Check sheet for the modelled part. Datum: model origin and axes. Units: mm. Face numbers are marked on the shaded views. A direction names the side the tool comes from. Give positions to 0.01 mm unless a question says otherwise; leave off trailing zeros. Order: outer loops, then holes, each group sorted by start corner. A loop starts at its lowest first (then second) coordinate and runs counter-clockwise, first axis right, second up. Notation, with made-up numbers: (-21, 35.5) - (-9, 35.5) arc R12 ccw to (-9, 52.5) - close; hole circle Ø4 at (58, 47). An arc over 180 degrees is marked (long way). Answer in a Markdown table with one row per item.
from build123d import *

# Parameters (mm, degrees)
SKETCH1_R           = 1.5
BOSS_EXTRUDE1_DEPTH = 3


with BuildPart() as part:
    # Sketch1 → Boss-Extrude1 (new body)
    with BuildSketch(Plane(origin=(0, 0, 0), x_dir=(1, 0, 0), z_dir=(0, 1, 0))):
        with BuildLine():
            Line((20.893657446, 4), (2.081641936, 4))
            ThreePointArc((2.081641936, 4), (2.861028333, 4.588201733), (3.521749436, 5.30713988))
            ThreePointArc((3.521749436, 5.30713988), (3.405395609, 5.596745198), (3.282888305, 5.883801663))
            ThreePointArc((3.282888305, 5.883801663), (1.93527598, 5.894040025), (0.627094961, 5.57027124))
            ThreePointArc((0.627094961, 5.57027124), (0.366286148, 6.046375), (0.084372603, 6.510293938))
            ThreePointArc((0.084372603, 6.510293938), (1.018855105, 7.48132754), (1.683794586, 8.65351323))
            ThreePointArc((1.683794586, 8.65351323), (1.496450048, 8.903135899), (1.303821399, 9.148703928))
            ThreePointArc((1.303821399, 9.148703928), (-0.000522033, 8.809805691), (-1.180330337, 8.158486898))
            ThreePointArc((-1.180330337, 8.158486898), (-1.555477026, 8.550865528), (-1.947855656, 8.926012217))
            ThreePointArc((-1.947855656, 8.926012217), (-1.296536862, 10.105820521), (-0.957638625, 11.410163953))
            ThreePointArc((-0.957638625, 11.410163953), (-1.203206655, 11.602792602), (-1.452829324, 11.79013714))
            ThreePointArc((-1.452829324, 11.79013714), (-2.625015014, 11.125197659), (-3.596048616, 10.190715157))
            ThreePointArc((-3.596048616, 10.190715157), (-4.059967554, 10.472628702), (-4.536071314, 10.733437515))
            ThreePointArc((-4.536071314, 10.733437515), (-4.212302529, 12.041618533), (-4.222540891, 13.389230859))
            ThreePointArc((-4.222540891, 13.389230859), (-4.509597355, 13.511738163), (-4.799202674, 13.62809199))
            ThreePointArc((-4.799202674, 13.62809199), (-5.759348103, 12.682425791), (-6.455432668, 11.528463019))
            ThreePointArc((-6.455432668, 11.528463019), (-6.976508546, 11.680699536), (-7.503891752, 11.809396783))
            ThreePointArc((-7.503891752, 11.809396783), (-7.529737283, 13.156800143), (-7.888414517, 14.455843809))
            ThreePointArc((-7.888414517, 14.455843809), (-8.197396993, 14.499881098), (-8.507248835, 14.537314892))
            ThreePointArc((-8.507248835, 14.537314892), (-9.18992168, 13.375367565), (-9.563620196, 12.080565177))
            ThreePointArc((-9.563620196, 12.080565177), (-10.106342554, 12.09275), (-10.649064912, 12.080565177))
            ThreePointArc((-10.649064912, 12.080565177), (-11.022763428, 13.375367565), (-11.705436272, 14.537314892))
            ThreePointArc((-11.705436272, 14.537314892), (-12.015288115, 14.499881098), (-12.324270591, 14.455843809))
            ThreePointArc((-12.324270591, 14.455843809), (-12.682947825, 13.156800143), (-12.708793355, 11.809396783))
            ThreePointArc((-12.708793355, 11.809396783), (-13.236176561, 11.680699536), (-13.757252439, 11.528463019))
            ThreePointArc((-13.757252439, 11.528463019), (-14.453337005, 12.682425791), (-15.413482434, 13.62809199))
            ThreePointArc((-15.413482434, 13.62809199), (-15.703087752, 13.511738163), (-15.990144217, 13.389230859))
            ThreePointArc((-15.990144217, 13.389230859), (-16.000382579, 12.041618533), (-15.676613793, 10.733437515))
            ThreePointArc((-15.676613793, 10.733437515), (-16.152717554, 10.472628702), (-16.616636492, 10.190715157))
            ThreePointArc((-16.616636492, 10.190715157), (-17.587670094, 11.125197659), (-18.759855783, 11.79013714))
            ThreePointArc((-18.759855783, 11.79013714), (-19.009478453, 11.602792602), (-19.255046482, 11.410163953))
            ThreePointArc((-19.255046482, 11.410163953), (-18.916148245, 10.105820521), (-18.264829452, 8.926012217))
            ThreePointArc((-18.264829452, 8.926012217), (-18.657208082, 8.550865528), (-19.032354771, 8.158486898))
            ThreePointArc((-19.032354771, 8.158486898), (-20.212163074, 8.809805691), (-21.516506507, 9.148703928))
            ThreePointArc((-21.516506507, 9.148703928), (-21.709135156, 8.903135899), (-21.896479694, 8.65351323))
            ThreePointArc((-21.896479694, 8.65351323), (-21.231540213, 7.48132754), (-20.297057711, 6.510293938))
            ThreePointArc((-20.297057711, 6.510293938), (-20.578971255, 6.046375), (-20.839780068, 5.57027124))
            ThreePointArc((-20.839780068, 5.57027124), (-22.147961087, 5.894040025), (-23.495573413, 5.883801663))
            ThreePointArc((-23.495573413, 5.883801663), (-23.618080717, 5.596745198), (-23.734434544, 5.30713988))
            ThreePointArc((-23.734434544, 5.30713988), (-22.788768345, 4.346994451), (-21.634805572, 3.650909885))
            ThreePointArc((-21.634805572, 3.650909885), (-21.78704209, 3.129834008), (-21.915739337, 2.602450802))
            ThreePointArc((-21.915739337, 2.602450802), (-23.263142697, 2.576605271), (-24.562186363, 2.217928037))
            ThreePointArc((-24.562186363, 2.217928037), (-24.606223651, 1.908945561), (-24.643657446, 1.599093719))
            ThreePointArc((-24.643657446, 1.599093719), (-23.481710119, 0.916420874), (-22.186907731, 0.542722358))
            ThreePointArc((-22.186907731, 0.542722358), (-22.199092554, 0), (-22.186907731, -0.542722358))
            ThreePointArc((-22.186907731, -0.542722358), (-23.481710119, -0.916420874), (-24.643657446, -1.599093719))
            ThreePointArc((-24.643657446, -1.599093719), (-24.606223651, -1.908945561), (-24.562186363, -2.217928037))
            ThreePointArc((-24.562186363, -2.217928037), (-23.263142697, -2.576605271), (-21.915739337, -2.602450802))
            ThreePointArc((-21.915739337, -2.602450802), (-21.78704209, -3.129834008), (-21.634805572, -3.650909885))
            ThreePointArc((-21.634805572, -3.650909885), (-22.788768345, -4.346994451), (-23.734434544, -5.30713988))
            ThreePointArc((-23.734434544, -5.30713988), (-23.618080717, -5.596745198), (-23.495573413, -5.883801663))
            ThreePointArc((-23.495573413, -5.883801663), (-22.147961087, -5.894040025), (-20.839780068, -5.57027124))
            ThreePointArc((-20.839780068, -5.57027124), (-20.578971255, -6.046375), (-20.297057711, -6.510293938))
            ThreePointArc((-20.297057711, -6.510293938), (-21.231540213, -7.48132754), (-21.896479694, -8.65351323))
            ThreePointArc((-21.896479694, -8.65351323), (-21.709135156, -8.903135899), (-21.516506507, -9.148703928))
            ThreePointArc((-21.516506507, -9.148703928), (-20.212163074, -8.809805691), (-19.032354771, -8.158486898))
            ThreePointArc((-19.032354771, -8.158486898), (-18.657208082, -8.550865528), (-18.264829452, -8.926012217))
            ThreePointArc((-18.264829452, -8.926012217), (-18.916148245, -10.105820521), (-19.255046482, -11.410163953))
            ThreePointArc((-19.255046482, -11.410163953), (-19.009478453, -11.602792602), (-18.759855783, -11.79013714))
            ThreePointArc((-18.759855783, -11.79013714), (-17.587670094, -11.125197659), (-16.616636492, -10.190715157))
            ThreePointArc((-16.616636492, -10.190715157), (-16.152717554, -10.472628702), (-15.676613793, -10.733437515))
            ThreePointArc((-15.676613793, -10.733437515), (-16.000382579, -12.041618533), (-15.990144217, -13.389230859))
            ThreePointArc((-15.990144217, -13.389230859), (-15.703087752, -13.511738163), (-15.413482434, -13.62809199))
            ThreePointArc((-15.413482434, -13.62809199), (-14.453337005, -12.682425791), (-13.757252439, -11.528463019))
            ThreePointArc((-13.757252439, -11.528463019), (-13.236176561, -11.680699536), (-12.708793355, -11.809396783))
            ThreePointArc((-12.708793355, -11.809396783), (-12.682947825, -13.156800143), (-12.324270591, -14.455843809))
            ThreePointArc((-12.324270591, -14.455843809), (-12.015288115, -14.499881098), (-11.705436272, -14.537314892))
            ThreePointArc((-11.705436272, -14.537314892), (-11.022763428, -13.375367565), (-10.649064912, -12.080565177))
            ThreePointArc((-10.649064912, -12.080565177), (-10.106342554, -12.09275), (-9.563620196, -12.080565177))
            ThreePointArc((-9.563620196, -12.080565177), (-9.18992168, -13.375367565), (-8.507248835, -14.537314892))
            ThreePointArc((-8.507248835, -14.537314892), (-8.197396993, -14.499881098), (-7.888414517, -14.455843809))
            ThreePointArc((-7.888414517, -14.455843809), (-7.529737283, -13.156800143), (-7.503891752, -11.809396783))
            ThreePointArc((-7.503891752, -11.809396783), (-6.976508546, -11.680699536), (-6.455432668, -11.528463019))
            ThreePointArc((-6.455432668, -11.528463019), (-5.759348103, -12.682425791), (-4.799202674, -13.62809199))
            ThreePointArc((-4.799202674, -13.62809199), (-4.509597355, -13.511738163), (-4.222540891, -13.389230859))
            ThreePointArc((-4.222540891, -13.389230859), (-4.212302529, -12.041618533), (-4.536071314, -10.733437515))
            ThreePointArc((-4.536071314, -10.733437515), (-4.059967554, -10.472628702), (-3.596048616, -10.190715157))
            ThreePointArc((-3.596048616, -10.190715157), (-2.625015014, -11.125197659), (-1.452829324, -11.79013714))
            ThreePointArc((-1.452829324, -11.79013714), (-1.203206655, -11.602792602), (-0.957638625, -11.410163953))
            ThreePointArc((-0.957638625, -11.410163953), (-1.296536862, -10.105820521), (-1.947855656, -8.926012217))
            ThreePointArc((-1.947855656, -8.926012217), (-1.555477026, -8.550865528), (-1.180330337, -8.158486898))
            ThreePointArc((-1.180330337, -8.158486898), (-0.000522033, -8.809805691), (1.303821399, -9.148703928))
            ThreePointArc((1.303821399, -9.148703928), (1.496450048, -8.903135899), (1.683794586, -8.65351323))
            ThreePointArc((1.683794586, -8.65351323), (1.018855105, -7.48132754), (0.084372603, -6.510293938))
            ThreePointArc((0.084372603, -6.510293938), (0.366286148, -6.046375), (0.627094961, -5.57027124))
            ThreePointArc((0.627094961, -5.57027124), (1.93527598, -5.894040025), (3.282888305, -5.883801663))
            ThreePointArc((3.282888305, -5.883801663), (3.405395609, -5.596745198), (3.521749436, -5.30713988))
            ThreePointArc((3.521749436, -5.30713988), (2.861028333, -4.588201733), (2.081641936, -4))
            Line((2.081641936, -4), (20.893657446, -4))
            ThreePointArc((20.893657446, -4), (24.893657446, 0), (20.893657446, 4))
        make_face()
        with Locations((-10.106342554, 0)):
            Circle(SKETCH1_R, mode=Mode.SUBTRACT)
        with Locations((20.893657446, 0)):
            Circle(SKETCH1_R, mode=Mode.SUBTRACT)
    extrude(amount=BOSS_EXTRUDE1_DEPTH)


solid = part.part
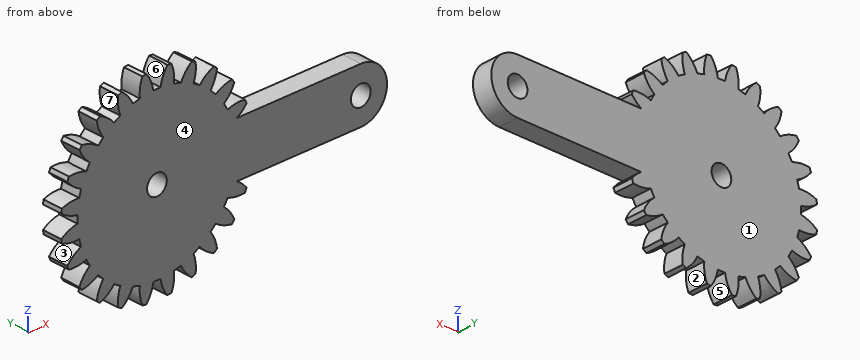
(1) Access from +Z, -Z, +X, -X, +Y, -Y to the whole of each face (thin tool, end or side, straight path). Record for the marked faces 1, 2 and 3.
Geometry says:
| item | result |
|---|---|
| face 1 | +Z, -Z, +X, -X, +Y |
| face 2 | +Y, -Y |
| face 3 | -X, +Y, -Y |
(2) Cross-section at B-B, the plane y = 0.9. Give the number of separate pieces and of enclosed holes in the cut face, then the cut area to 3 significant figures.
Geometry says:
| item | result |
|---|---|
| separate pieces | 1 |
| enclosed holes | 2 |
| area | 712 mm² |
(3) Thickness scan on L1, parallel to X at y = 1.15, z = 0; L2, parallel to Z at x = -21, y = 0.4; L3, parallel to Z at x = -22, y = 1.05. Record the ranges inside material, lowest first.
Geometry says:
| item | result |
|---|---|
| L1 | -22.2 to -11.61, -8.61 to 19.39, 22.39 to 24.89 |
| L2 | -9.06 to -7.19, -5.63 to 5.63, 7.19 to 9.06 |
| L3 | -5.87 to -3.83, -2.61 to 2.61, 3.83 to 5.87 |
(4) Gauge pin test, flat ends, axial feed: P1, Ø1.5, axis at x = 7, y = 2, coming from the +Z side; P2, Ø0.9, axis at x = 14, y = 1, coming from the -Z side; P3, Ø1.5, axis at y = 2, z = 8.5, coming from the +X side; P4, Ø1.8, axis at x = 20.89, z = 0, coming from the +Y side. Record the tip position at first contact, or that the pin passes through.
Geometry says:
| item | result |
|---|---|
| P1 | z = 4 |
| P2 | z = -4 |
| P3 | x = 1.68 |
| P4 | through |
(5) Cross-section at A-A, the plane z = 0. Record the cut outline in (x, y), then the cut area to 3 significant figures.
Geometry says:
| item | result |
|---|---|
| outline | (-22.2, 0) - (-11.61, 0) - (-11.61, 3) - (-22.2, 3) - close; (-8.61, 0) - (19.39, 0) - (19.39, 3) - (-8.61, 3) - close; (22.39, 0) - (24.89, 0) - (24.89, 3) - (22.39, 3) - close |
| area | 123 mm² |
(6) Cross-section at D-D, the plane z = -7.5. Record the cut outline in (x, y), then the cut area to 3 significant figures.
Geometry says:
| item | result |
|---|---|
| outline | (-21.25, 0) - (1.03, 0) - (1.03, 3) - (-21.25, 3) - close |
| area | 66.8 mm² |
(7) Cross-section at C-C, the plane z = 7. Record the cut outline in (x, y).
Geometry says:
| item | result |
|---|---|
| outline | (-20.83, 0) - (0.61, 0) - (0.61, 3) - (-20.83, 3) - close |
(8) Mould release check, pull along Z, two halves, no side actions. Record for the marked faces 4, 5, 6 and 7: pulls with the +Z half, pulls with the -Z half, needs draft (parallel to the pull), parting line crosses it, or undercut.
Geometry says:
| item | result |
|---|---|
| face 4 | needs draft |
| face 5 | pulls with the -Z half |
| face 6 | pulls with the +Z half |
| face 7 | undercut |
